Source: CAD feature listing. Evaluate the final solid. Frame: model axes, mm. Face numbers are marked on the shaded views. A direction names the side the tool comes from. Give positions to 0.01 mm unless a question says otherwise; leave off trailing zeros. Order: outer loops, then holes, each group sorted by start corner. A loop starts at its lowest first (then second) coordinate and runs counter-clockwise, first axis right, second up. Notation, with made-up numbers: (1.25, 43.25) - (60.25, 43.25) arc R15 ccw to (60.25, 64.25) - close; hole circle Ø9 at (78, -3.5). An arc over 180 degrees is marked (long way). Answer as CSV lines item,"result".
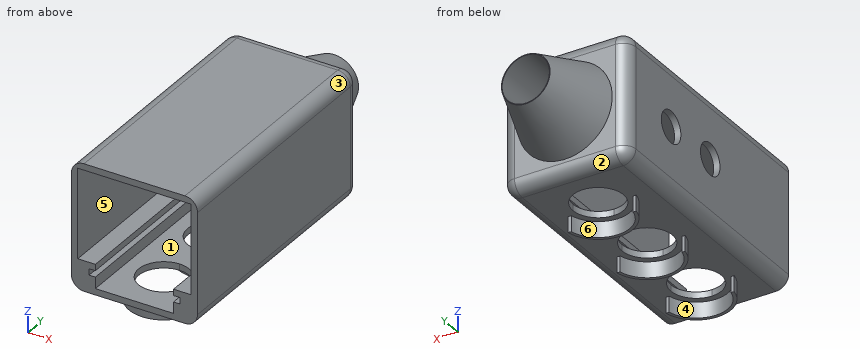
```python
from build123d import *

# Parameters (mm, degrees)
F0_W      = 50.8
F0_H      = 50.8
F1_DEPTH  = 101.6
F3_DEPTH  = 7.62
F5_DEPTH  = 7.62
F7_DEPTH  = 6.35
F8_W      = 50.8
F8_H      = 50.8
F9_DEPTH  = 2.54
F11_DEPTH = 25.4
F11_TAPER = 20
F12_R     = 9.525
F13_DEPTH = 129.541
F14_R     = 5.08


with BuildPart() as f1:
    # F0 (on Front) → F1 (new body)
    with BuildSketch(Plane.XZ):
        with Locations((25.4, 25.4)):
            Rectangle(F0_W, F0_H)
        Polygon((2.54, 12.192), (2.54, 48.26), (48.26, 48.26), (48.26, 12.192), (41.148, 12.192), (41.148, 9.652), (43.688, 9.652), (43.688, 7.112), (41.148, 7.112), (41.148, 2.54), (9.652, 2.54), (9.652, 7.112), (7.112, 7.112), (7.112, 9.652), (9.652, 9.652), (9.652, 12.192), align=None, mode=Mode.SUBTRACT)
    extrude(amount=F1_DEPTH)

    # F2 (on face) → F3 (cut)
    with BuildSketch(Plane(origin=(0, 0, 0), x_dir=(1, 0, 0), z_dir=(0, 0, -1))):
        with BuildLine():
            ThreePointArc((25.4, 8.89), (32.5842048969, 11.8657951031), (35.56, 19.05))
            ThreePointArc((35.56, 19.05), (32.5842048969, 26.2342048969), (25.4, 29.21))
            Line((25.4, 29.21), (25.4, 8.89))
        make_face()
        with BuildLine():
            Line((25.4, 8.89), (25.4, 29.21))
            ThreePointArc((25.4, 29.21), (15.24, 19.05), (25.4, 8.89))
        make_face()
        with BuildLine():
            Line((25.4, 60.96), (25.4, 40.64))
            ThreePointArc((25.4, 40.64), (32.5842048969, 43.6157951031), (35.56, 50.8))
            ThreePointArc((35.56, 50.8), (32.5842048969, 57.9842048969), (25.4, 60.96))
        make_face()
        with BuildLine():
            ThreePointArc((25.4, 60.96), (15.24, 50.8), (25.4, 40.64))
            Line((25.4, 40.64), (25.4, 60.96))
        make_face()
        with BuildLine():
            Line((25.4, 92.71), (25.4, 72.39))
            ThreePointArc((25.4, 72.39), (32.5842048969, 75.3657951031), (35.56, 82.55))
            ThreePointArc((35.56, 82.55), (32.5842048969, 89.7342048969), (25.4, 92.71))
        make_face()
        with BuildLine():
            ThreePointArc((25.4, 92.71), (15.24, 82.55), (25.4, 72.39))
            Line((25.4, 72.39), (25.4, 92.71))
        make_face()
    extrude(amount=-F3_DEPTH, mode=Mode.SUBTRACT)

    # F4 (on face) → F5 (cut)
    with BuildSketch(Plane(origin=(0, 0, 0), x_dir=(0, -1, 0), z_dir=(-1, 0, 0))):
        with BuildLine():
            Line((44.45, 25.4), (57.15, 25.4))
            ThreePointArc((57.15, 25.4), (50.8, 31.75), (44.45, 25.4))
        make_face()
        with BuildLine():
            ThreePointArc((19.05, 25.4), (25.4, 19.05), (31.75, 25.4))
            Line((31.75, 25.4), (19.05, 25.4))
        make_face()
        with BuildLine():
            Line((19.05, 25.4), (31.75, 25.4))
            ThreePointArc((31.75, 25.4), (25.4, 31.75), (19.05, 25.4))
        make_face()
        with BuildLine():
            ThreePointArc((44.45, 25.4), (50.8, 19.05), (57.15, 25.4))
            Line((57.15, 25.4), (44.45, 25.4))
        make_face()
    extrude(amount=-F5_DEPTH, mode=Mode.SUBTRACT)

    # F6 (on face) → F7 (join)
    with BuildSketch(Plane(origin=(0, 0, 0), x_dir=(1, 0, 0), z_dir=(0, 0, -1))):
        with BuildLine():
            ThreePointArc((12.9565921067, 85.09), (25.4, 95.25), (37.8434078933, 85.09))
            Line((37.8434078933, 85.09), (39.1371503595, 85.09))
            ThreePointArc((39.1371503595, 85.09), (25.4, 96.52), (11.6628496405, 85.09))
            Line((11.6628496405, 85.09), (12.9565921067, 85.09))
        make_face()
        with BuildLine():
            ThreePointArc((12.9565921067, 53.34), (25.4, 63.5), (37.8434078933, 53.34))
            Line((37.8434078933, 53.34), (39.1371503595, 53.34))
            ThreePointArc((39.1371503595, 53.34), (25.4, 64.77), (11.6628496405, 53.34))
            Line((11.6628496405, 53.34), (12.9565921067, 53.34))
        make_face()
        with BuildLine():
            ThreePointArc((12.9565921067, 21.59), (25.4, 31.75), (37.8434078933, 21.59))
            Line((37.8434078933, 21.59), (39.1371503595, 21.59))
            ThreePointArc((39.1371503595, 21.59), (25.4, 33.02), (11.6628496405, 21.59))
            Line((11.6628496405, 21.59), (12.9565921067, 21.59))
        make_face()
    extrude(amount=F7_DEPTH)

    # F8 (on face) → F9 (join)
    with BuildSketch(Plane(origin=(0, 0, 0), x_dir=(-1, 0, 0), z_dir=(0, 1, 0))):
        with Locations((-25.4, 25.4)):
            Rectangle(F8_W, F8_H)
    extrude(amount=F9_DEPTH)

    # F10 (on face) → F11 (join)
    with BuildSketch(Plane(origin=(0, 2.54, 0), x_dir=(-1, 0, 0), z_dir=(0, 1, 0))):
        with BuildLine():
            Line((-44.45, 25.4), (-6.35, 25.4))
            ThreePointArc((-6.35, 25.4), (-25.4, 44.45), (-44.45, 25.4))
        make_face()
        with BuildLine():
            ThreePointArc((-44.45, 25.4), (-25.4, 6.35), (-6.35, 25.4))
            Line((-6.35, 25.4), (-44.45, 25.4))
        make_face()
    extrude(amount=F11_DEPTH, taper=F11_TAPER)

    # F12 (on face) → F13 (cut, through all)
    with BuildSketch(Plane(origin=(0, 27.94, 0), x_dir=(-1, 0, 0), z_dir=(0, 1, 0))):
        with Locations((-25.4, 25.4)):
            Circle(F12_R)
    extrude(amount=-F13_DEPTH, mode=Mode.SUBTRACT)

    # F14
    f14_edges = [f1.edges().sort_by_distance(p)[0] for p in [
        (25.4, 2.54, 0),
        (0, 2.54, 25.4),
        (0, -49.53, 0),
        (50.8, -49.53, 0),
        (50.8, 2.54, 25.4),
        (25.4, 2.54, 50.8),
        (50.8, -49.53, 50.8),
        (0, -49.53, 50.8),
    ]]
    fillet(f14_edges, radius=F14_R)


solid = f1.part
```
(1) Ray query, line 1 (X direction, y = -15, z = 21); line 2 (Y direction, x = 1, z = 25). Return the intervals inside material, ascending. Write a range as from..to.
Completed:
line 1,"0..2.54, 48.26..50.8"
line 2,"-101.6..-57.14, -44.46..-31.74, -19.06..0.49"
(2) Contact query for flat-ended pins moving along their axis: pin 1 (3 mm diameter, centred on x = 40, y = -76.5, fed in from -Z); pin 2 (10 mm diameter, centred on x = 22.5, z = 31, fed in from +Y); pin 3 (13.5 mm diameter, centred on x = 29.5, z = 28, fed in from -Y); pin 4 (1.5 mm diameter, centred on y = -15, z = 0, fed in from +X). Output: stop coordinate, or through.
Completed:
pin 1,"z = 0"
pin 2,"y = 27.94"
pin 3,"y = 0"
pin 4,"x = 48.38"
(3) Cut plane D-D (y = 18.5). Return loops of the section in (x, z) (3 decimals), then the cut area to 3 significant figures.
Completed:
outline,"circle Ø26.482 at (25.4, 25.4); hole circle Ø19.05 at (25.4, 25.4)"
area,"266 mm²"
(4) Cut plane B-B (z = 25.4). Give the number of separate pieces and of enclosed holes in the cut face, then the cut area to 3 significant figures.
Completed:
separate pieces,"4"
enclosed holes,"0"
area,"770 mm²"
(5) Mould query, pull axis X, two halves, no side actions, for the marked faces 1, 2 and 3. Classes: released by +X, released by -X, zero draft, split by the parting line, or undercut.
Completed:
face 1,"undercut"
face 2,"zero draft"
face 3,"released by +X"
(6) Cut plane C-C (y = -79). Return loops of the section in (x, z).
Completed:
outline,"(0, 5.08) arc R5.08 ccw to (5.08, 0) - (15.88, 0) - (15.88, 2.54) - (9.65, 2.54) - (9.65, 7.11) - (7.11, 7.11) - (7.11, 9.65) - (9.65, 9.65) - (9.65, 12.19) - (2.54, 12.19) - (2.54, 48.26) - (48.26, 48.26) - (48.26, 12.19) - (41.15, 12.19) - (41.15, 9.65) - (43.69, 9.65) - (43.69, 7.11) - (41.15, 7.11) - (41.15, 2.54) - (34.92, 2.54) - (34.92, 0) - (45.72, 0) arc R5.08 ccw to (50.8, 5.08) - (50.8, 45.72) arc R5.08 ccw to (45.72, 50.8) - (5.08, 50.8) arc R5.08 ccw to (0, 45.72) - close"
(7) Access query for the marked faces 4, 5 and 6. Directions: +Z, -Z, +X, -X, +Y, -Y. A direction counts if a zero-diameter tool reaches every point of the face in a straight line with its end or side. Return the directions, or none.
Completed:
face 4,"-Z"
face 5,"-Y"
face 6,"-Z, +Y"
(8) Cut plane A-A (y = -38). Return loops of the section in (x, z).
Completed:
outline,"(0, 5.08) arc R5.08 ccw to (5.08, 0) - (45.72, 0) arc R5.08 ccw to (50.8, 5.08) - (50.8, 45.72) arc R5.08 ccw to (45.72, 50.8) - (5.08, 50.8) arc R5.08 ccw to (0, 45.72) - close; hole (2.54, 12.19) - (9.65, 12.19) - (9.65, 9.65) - (7.11, 9.65) - (7.11, 7.11) - (9.65, 7.11) - (9.65, 2.54) - (41.15, 2.54) - (41.15, 7.11) - (43.69, 7.11) - (43.69, 9.65) - (41.15, 9.65) - (41.15, 12.19) - (48.26, 12.19) - (48.26, 48.26) - (2.54, 48.26) - close"
